Geometry: see drawing. Coordinates: mm, zero at the bounding-box minimum. A direction names the side the tool comes from. Give positions to 0.01 mm unless a question says otherwise; leave off trailing zeros. Loops run counter-clockwise (first coordinate to the right, second up) from the corner with the lowest first, then second, coordinate; pieces in that order, holes last. Notation, with made-up numbers: (-33.75, 64) -> (21.25, 64) arc R32 cw to (21.25, 96) -> close; hole circle Ø7 at (49, 19). An arc over 180 degrees is marked (long way). Use CSV: the item, a comma, the result in double quotes.
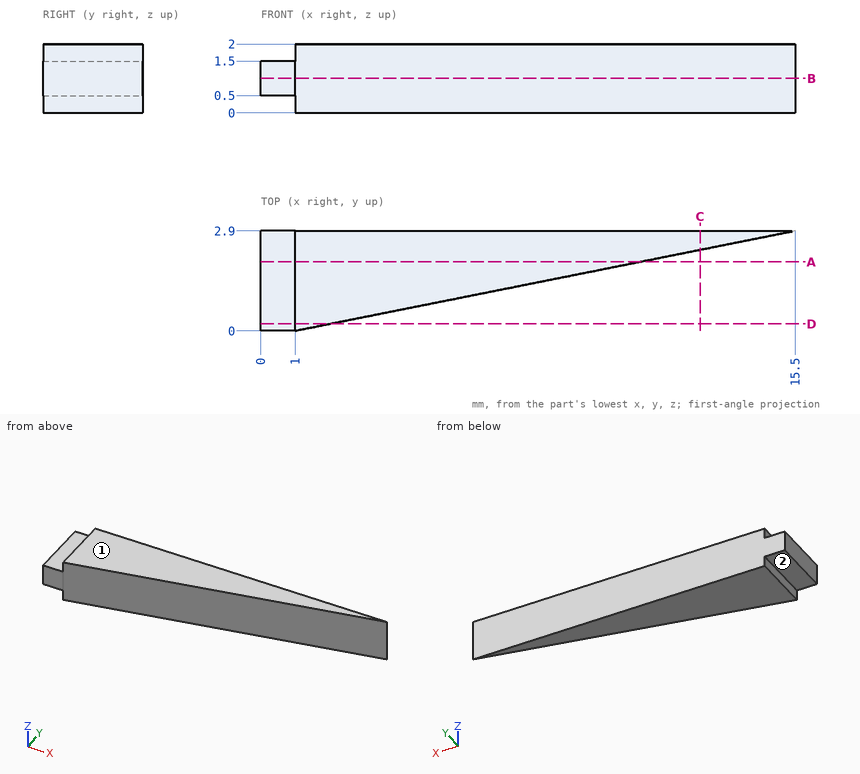
1) Reachability of the marked faces 1 and 2 from +Z, -Z, +X, -X, +Y, -Y: full face, straight path, thin tool, end or side. Return the list, or none.
From the geometry:
face 1,"+Z, +X, -X, +Y, -Y"
face 2,"-Z, -X, +Y, -Y"
2) Section query C-C (x = 12.75). Return loops of the section in (y, z).
From the geometry:
outline,"(2.35, 0) -> (2.9, 0) -> (2.9, 2) -> (2.35, 2) -> close"
3) Contact query for a flat-ended pin moving along its axis: pin 1 (1 mm diameter, centred on x = 11.5, y = 1.5, fed in from +Z). Output: stop coordinate, or through.
From the geometry:
pin 1,"passes through"
4) Ray query, line 1 (Y direction, x = 11, z = 0.9); line 2 (Z direction, x = 0.75, y = 1.75); line 3 (Y direction, x = 2, z = 0.9). Return the intervals inside material, ascending.
From the geometry:
line 1,"y = 2 to 2.9"
line 2,"z = 0.5 to 1.5"
line 3,"y = 0.2 to 2.9"
5) Section query A-A (y = 2). Return loops of the section in (x, z).
From the geometry:
outline,"(0, 0.5) -> (1, 0.5) -> (1, 0) -> (11, 0) -> (11, 2) -> (1, 2) -> (1, 1.5) -> (0, 1.5) -> close"
6) Section query B-B (z = 1). Return loops of the section in (x, y).
From the geometry:
outline,"(0, 0) -> (1, 0) -> (15.5, 2.9) -> (0, 2.9) -> close"
7) Section query D-D (y = 0.2). Return loops of the section in (x, z), then the cut area to 3 significant figures.
From the geometry:
outline,"(0, 0.5) -> (1, 0.5) -> (1, 0) -> (2, 0) -> (2, 2) -> (1, 2) -> (1, 1.5) -> (0, 1.5) -> close"
area,"3.00 mm^2"
